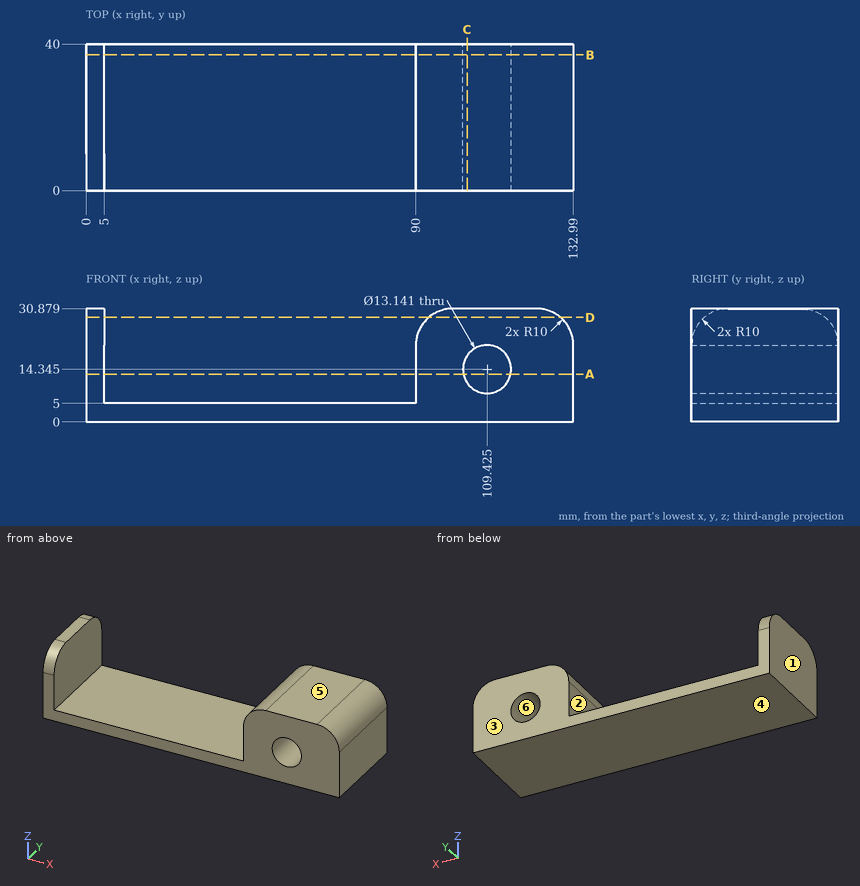
Drawing for the job (mm, zero at the part's lowest x, y, z). A direction names the side the tool comes from. Give positions to 0.01 mm unless a question says otherwise; leave off trailing zeros. Order: outer loops, then holes, each group sorted by start corner. A loop starts at its lowest first (then second) coordinate and runs counter-clockwise, first axis right, second up. Notation, with made-up numbers: (86, 17) - (105, 17) arc R22 cw to (105, 36) - close; hole circle Ø4 at (73, 77). An arc over 180 degrees is marked (long way). Write item = value, one per line. Start each with the question number.
1. Two-plate mould, pull along Z, no slides. Class the marked faces 3, 4, 5 and 6: pulls with the +Z half, pulls with the -Z half, needs draft (parallel to the pull), parting line crosses it, or undercut.
2. Probe line 1 along X through (y, z) = (15, 11.5); line 2 along X through (y, z) = (14.5, 18.5) (1 decimal); line 3 along Z through (x, y) = (31, 30). List the from-to ranges inside material, lowest first.
3. Cut at C-C, the plane x = 104. List the corners of the cut face in (y, z).
4. Cut at B-B, the plane y = 37. List the corners of the cut face in (x, z) (1 decimal), and give its area (3 significant figures).
5. Drop flat-ended pins along their axis: P1, Ø10, axis at x = 87, y = 18, coming from the +Z side; P2, Ø3, axis at y = 23, z = 27, coming from the +X side; P3, Ø20, axis at x = 43, y = 19.5, coming from the +Z side. Give the stop position or say it passes through.
6. Which spindle directions (+Z, -Z, +X, -X, +Y, -Y) get a long thin tool onto all of the face, cutting with end or side? Do the marked faces 1 and 2. Say none if no direction does.
7. Cut at A-A, the plane z = 13. List the corners of the cut face in (x, y), and give its area (4 significant figures).
8. Cut at D-D, the plane z = 28.5. List the corners of the cut face in (x, y) (1 decimal).
Taken from the geometry:
q1.face_3 = needs draft
q1.face_4 = pulls with the -Z half
q1.face_5 = pulls with the +Z half
q1.face_6 = undercut
q2.line_1 = 0 to 5, 90 to 103.5, 115.35 to 132.99
q2.line_2 = 0 to 5, 90 to 104.3, 114.5 to 133
q2.line_3 = 0 to 5
q3.outline = (0, 0) - (40, 0) - (40, 10.64) - (0, 10.64) - close; (0, 18.05) - (40, 18.05) - (40, 30.88) - (0, 30.88) - close
q4.outline = (0, 0) - (133, 0) - (133, 20.9) arc R10 ccw to (123, 30.9) - (100, 30.9) arc R10 ccw to (90, 20.9) - (90, 5) - (5, 5) - (5, 28) - (0, 28) - close; hole circle Ø13.1 at (109.4, 14.3)
q4.area = 1,710 mm²
q5.P1 = 26.88
q5.P2 = 131.86
q5.P3 = 5
q6.face_1 = +Z, -Z, -X, +Y, -Y
q6.face_2 = +Z, +Y, -Y
q7.outline = (0, 0) - (5, 0) - (5, 40) - (0, 40) - close; (90, 0) - (102.99, 0) - (102.99, 40) - (90, 40) - close; (115.86, 0) - (132.99, 0) - (132.99, 40) - (115.86, 40) - close
q7.area = 1,405 mm²
q8.outline = (0, 3.5) - (5, 3.5) - (5, 36.5) - (0, 36.5) - close; (93.5, 0) - (129.5, 0) - (129.5, 40) - (93.5, 40) - close
